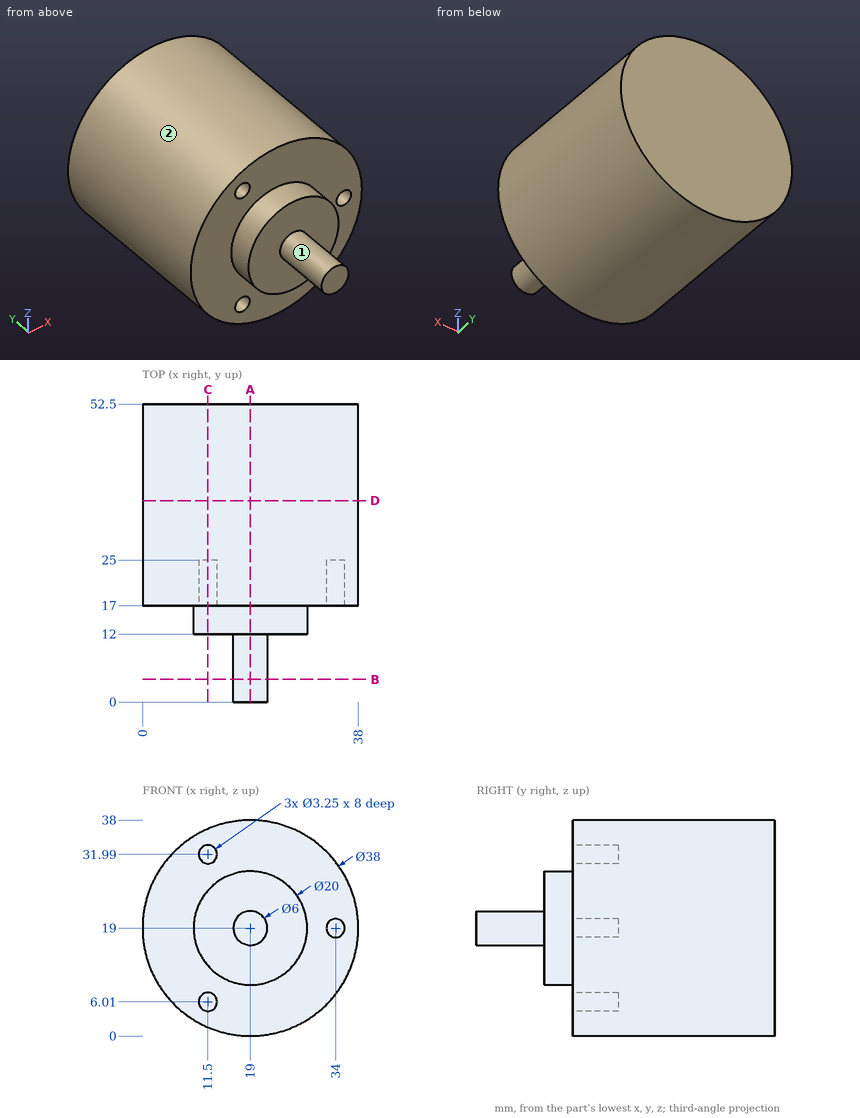
Answer from the drawing. Dimensions are ordinates in mm from the lowest x, y and z of the part. A direction names the side the tool comes from. Round coordinates to 2 decimals unless told otherwise and drop trailing zeros. Write each loop counter-clockwise with the first axis right and the second up, starting at its lowest first coordinate (ties: lowest second). Pieces come first, ordered by that corner, then holes. Notation, with made-up numbers: M -5.75,-4 L 33.25,-4 A26 ccw 33.25,29 Z; hole C -27,81.25 d2. An arc over 180 degrees is marked long. Write each question's results on one line, items separated by ' | '. Start each with the question number.
Item 1: Find section A-A on x = 19. Write down the section's boundary in (y, z).
Item 2: Find section D-D on y = 35.5. Write down the section's boundary in (x, z), and give its area (3 significant figures).
Item 3: Which of the six approach directions +Z, -Z, +X, -X, +Y, -Y give full straight-line access (tool end or side, diameter ignored) to the marked faces 1 and 2?
Item 4: Find section C-C on x = 11.5. Write down the section's boundary in (y, z) (1 decimal), and give its area (3 significant figures).
Item 5: Straight lines are drawn through the part: probe 1 along Z at (x, y) = (11.5, 19.25) (1 decimal); probe 2 along Y at (x, z) = (2, 27); probe 3 along Y at (x, z) = (18, 11). For each, find the intervals that lie inside material, in ascending order.
Item 6: Given pin 1 Ø1.5 at (x, y) = (28.5, 28.5) entering from +Z (1 decimal); pin 2 Ø2 at (y, z) = (16.5, 15) entering from +X; pin 3 Ø3 at (x, z) = (11.5, 31.99) entering from -Y, each flat-ended and moving along its own axis, determine where each tip first touches the part or whether it passes through.
Item 7: Find section B-B on y = 4. Write down the section's boundary in (x, z).
Answer block:
1) outline: M 0,16 L 12,16 L 12,9 L 17,9 L 17,0 L 52.5,0 L 52.5,38 L 17,38 L 17,29 L 12,29 L 12,22 L 0,22 Z
2) outline: C 19,19 d38 | area: 1,130 mm²
3) face 1: -Y | face 2: +Y, -Y
4) outline: M 12,12.4 L 17,12.4 L 17,7.6 L 25,7.6 L 25,4.4 L 17,4.4 L 17,1.5 L 52.5,1.5 L 52.5,36.5 L 17,36.5 L 17,33.6 L 25,33.6 L 25,30.4 L 17,30.4 L 17,25.6 L 12,25.6 Z | area: 1,250 mm²
5) probe 1: z = 1.5 to 4.4, 7.6 to 30.4, 33.6 to 36.5 | probe 2: y = 17 to 52.5 | probe 3: y = 12 to 52.5
6) pin 1: stops at z = 35.9 | pin 2: stops at x = 37.74 | pin 3: stops at y = 25
7) outline: C 19,19 d6
